from build123d import *

# Parameters (mm, degrees)
SKETCH1_W           = 50
SKETCH1_H           = 70
SKETCH1_R           = 1.5
BOSS_EXTRUDE1_DEPTH = 5
SKETCH2_W           = 5
SKETCH2_H           = 70
BOSS_EXTRUDE2_DEPTH = 40
FILLET1_R           = 30
CUT_EXTRUDE1_DEPTH  = 51


with BuildPart() as part:
    # Sketch1 → Boss-Extrude1 (new body)
    with BuildSketch(Plane(origin=(0, 0, 0), x_dir=(1, 0, 0), z_dir=(0, 1, 0))):
        with Locations((-195.719432441, 94.934599156)):
            Rectangle(SKETCH1_W, SKETCH1_H)
        with Locations((-185.719432441, 94.934599156)):
            Circle(SKETCH1_R, mode=Mode.SUBTRACT)
        with Locations((-205.719432441, 94.934599156)):
            Circle(SKETCH1_R, mode=Mode.SUBTRACT)
        with Locations((-205.719432441, 104.934599156)):
            Circle(SKETCH1_R, mode=Mode.SUBTRACT)
        with Locations((-185.719432441, 104.934599156)):
            Circle(SKETCH1_R, mode=Mode.SUBTRACT)
        with Locations((-205.719432441, 114.934599156)):
            Circle(SKETCH1_R, mode=Mode.SUBTRACT)
        with Locations((-185.719432441, 114.934599156)):
            Circle(SKETCH1_R, mode=Mode.SUBTRACT)
        with Locations((-205.719432441, 124.934599156)):
            Circle(SKETCH1_R, mode=Mode.SUBTRACT)
        with Locations((-185.719432441, 124.934599156)):
            Circle(SKETCH1_R, mode=Mode.SUBTRACT)
        with Locations((-205.719432441, 84.934599156)):
            Circle(SKETCH1_R, mode=Mode.SUBTRACT)
        with Locations((-185.719432441, 84.934599156)):
            Circle(SKETCH1_R, mode=Mode.SUBTRACT)
        with Locations((-205.719432441, 74.934599156)):
            Circle(SKETCH1_R, mode=Mode.SUBTRACT)
        with Locations((-185.719432441, 74.934599156)):
            Circle(SKETCH1_R, mode=Mode.SUBTRACT)
        with Locations((-205.719432441, 64.934599156)):
            Circle(SKETCH1_R, mode=Mode.SUBTRACT)
        with Locations((-185.719432441, 64.934599156)):
            Circle(SKETCH1_R, mode=Mode.SUBTRACT)
        with BuildLine():
            Line((-197.219432441, 124.934599156), (-197.219432441, 64.934599156))
            ThreePointArc((-197.219432441, 64.934599156), (-195.719432441, 63.434599156), (-194.219432441, 64.934599156))
            Line((-194.219432441, 64.934599156), (-194.219432441, 124.934599156))
            ThreePointArc((-194.219432441, 124.934599156), (-195.719432441, 126.434599156), (-197.219432441, 124.934599156))
        make_face(mode=Mode.SUBTRACT)
    extrude(amount=BOSS_EXTRUDE1_DEPTH)

    # Sketch2 → Boss-Extrude2 (add)
    with BuildSketch(Plane(origin=(0, 0, 0), x_dir=(1, 0, 0), z_dir=(0, 1, 0))):
        with Locations((-218.219432441, 94.934599156)):
            Rectangle(SKETCH2_W, SKETCH2_H)
        with Locations((-173.219432441, 94.934599156)):
            Rectangle(SKETCH2_W, SKETCH2_H)
    extrude(amount=-BOSS_EXTRUDE2_DEPTH)

    # Fillet1
    fillet1_edges = [part.edges().sort_by_distance(p)[0] for p in [
        (-218.219432441, -40, -129.934599156),
        (-218.219432441, -40, -59.934599156),
        (-173.219432441, -40, -59.934599156),
        (-173.219432441, -40, -129.934599156),
    ]]
    fillet(fillet1_edges, radius=FILLET1_R)

    # Sketch3 → Cut-Extrude1 (cut, through all)
    with BuildSketch(Plane(origin=(-170.719432441, 0, 0), x_dir=(0, 0, -1), z_dir=(1, 0, 0))):
        with BuildLine():
            Line((94.934599156, -27), (96.434599156, -27))
            Line((96.434599156, -27), (96.434599156, -28.034196172))
            ThreePointArc((96.434599156, -28.034196172), (94.934599156, -36.24), (93.434599156, -28.034196172))
            Line((93.434599156, -28.034196172), (93.434599156, -27))
            Line((93.434599156, -27), (94.934599156, -27))
        make_face()
    extrude(amount=-CUT_EXTRUDE1_DEPTH, mode=Mode.SUBTRACT)


solid = part.part
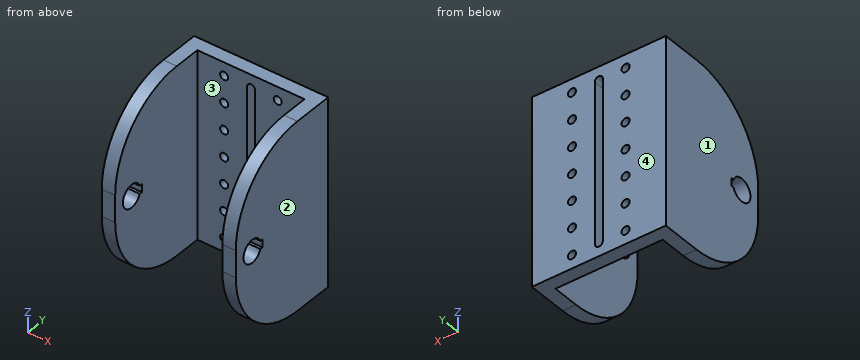
Here's how the part is built. I have some questions about the finished solid (model axes, mm). Face numbers are marked on the shaded views. Coordinates: 2 decimals unless noted, no trailing zeros. Loops run counter-clockwise (first coordinate to the right, second up) from the corner with the lowest first, then second, coordinate; pieces in that order, holes last. Notation, with made-up numbers: (81, 10.25) -> (134, 10.25) arc R30 cw to (134, 48.25) -> close; hole circle Ø9 at (-5.75, 81.25). An arc over 180 degrees is marked (long way). Use one line per item in the form item = value. Start each with the question number.
(1) Please list where these lines run through material, in increasing order: line 1 along X through (y, z) = (-34.5, -109.5); line 2 along Y through (x, z) = (-217.5, -93); line 3 along Y through (x, z) = (-206, -70.5).
(2) If we section it at D-D (x = -208.5): Please give me the cut outline in (y, z), then the cut area to 3 significant figures.
(3) If we section it at B-B (z = -112.5): Please give me the cut outline in (x, y).
(4) Will these pins go through, and if not, where does the flat tip stop? pin 1 (1.1 mm diameter, centred on x = -217.5, y = -27.5, fed in from +Z); pin 2 (5 mm diameter, centred on y = -32, z = -94.93, fed in from -X); pin 3 (1.5 mm diameter, centred on x = -185.5, z = -110.5, fed in from -Y).
(5) We'd pull the mould along X, two halves only. Please class the marked faces 1, 2, 3 and 4: pulls with the +X half, pulls with the -X half, needs draft (parallel to the pull), parting line crosses it, or undercut.
(6) If we section it at C-C (y = -32): Please give me the cut outline in (x, z), then the cut area to 3 significant figures.
(7) If we section it at A-A (y = -19.5): Please give me the cut outline in (x, z).
Verdict:
q1.line_1 = -220.72 to -215.72, -175.72 to -170.72
q1.line_2 = -40 to -35.77, -28.23 to 5
q1.line_3 = 0 to 5
q2.outline = (0, -129.93) -> (5, -129.93) -> (5, -59.93) -> (0, -59.93) -> close
q2.area = 350 mm²
q3.outline = (-220.72, -37.24) -> (-215.72, -37.24) -> (-215.72, 0) -> (-197.22, 0) -> (-197.22, 5) -> (-220.72, 5) -> close; (-194.22, 0) -> (-175.72, 0) -> (-175.72, -37.24) -> (-170.72, -37.24) -> (-170.72, 5) -> (-194.22, 5) -> close
q4.pin_1 = -65.18
q4.pin_2 = through
q4.pin_3 = 0
q5.face_1 = pulls with the -X half
q5.face_2 = pulls with the +X half
q5.face_3 = undercut
q5.face_4 = needs draft
q6.outline = (-220.72, -120.33) -> (-215.72, -120.33) -> (-215.72, -99.17) -> (-220.72, -99.17) -> close; (-220.72, -90.69) -> (-215.72, -90.69) -> (-215.72, -69.54) -> (-220.72, -69.54) -> close; (-175.72, -120.33) -> (-170.72, -120.33) -> (-170.72, -99.17) -> (-175.72, -99.17) -> close; (-175.72, -90.69) -> (-170.72, -90.69) -> (-170.72, -69.54) -> (-175.72, -69.54) -> close
q6.area = 423 mm²
q7.outline = (-220.72, -128.39) -> (-215.72, -128.39) -> (-215.72, -61.48) -> (-220.72, -61.48) -> close; (-175.72, -128.39) -> (-170.72, -128.39) -> (-170.72, -61.48) -> (-175.72, -61.48) -> close
